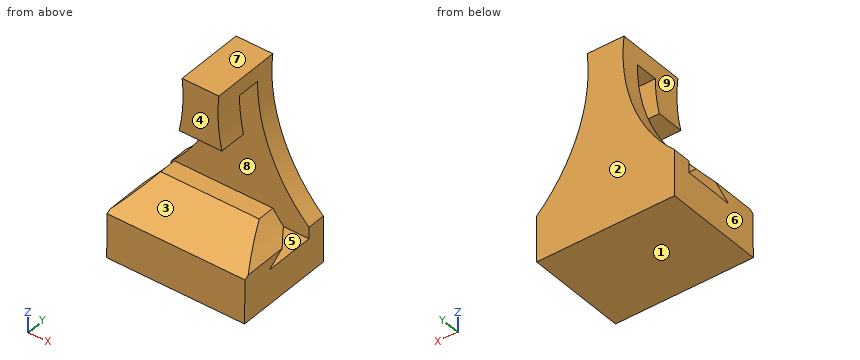
```python
from build123d import *

# Parameters (mm, degrees)
F1_DEPTH = 60
F3_DEPTH = 43.8751131995


# Not quite as in the source:
# - a pattern or mirror of a feature is missing from the dataset's text; its kind, count and spacing are read off the source's solid


with BuildPart() as f1:
    # F0 (on Right) → F1 (new body)
    with BuildSketch(Plane.YZ):
        Polygon((-43.8741131995, 0), (0, 0), (0, 80), (-30, 80), (-30, 56.7161887884), (-18, 56.7161887884), (-18, 72.701357305), (-8, 72.701357305), (-8, 15), (-30, 15), (-17.1229156852, 24.1054718941), (-17.1229156852, 29.8044607043), (-24.7526019812, 29.8044607043), (-43.619140311, 18.9982891026), align=None)
    extrude(amount=F1_DEPTH)

    # F2 (on face) → F3 (cut, through all)
    with BuildSketch(Plane(origin=(0, 0, 0), x_dir=(-1, 0, 0), z_dir=(0, 1, 0))):
        with BuildLine():
            Line((-60, 80), (-60, 20))
            ThreePointArc((-60, 20), (-42.0220624026, 47.4414228809), (-38, 80))
            Line((-38, 80), (-60, 80))
        make_face()
    f3 = extrude(amount=-F3_DEPTH, mode=Mode.SUBTRACT)

    # F3_copies: F3 across plane
    add(f3.mirror(Plane(origin=(30, 0, 0), x_dir=(0, 0, -1), z_dir=(-1, 0, 0))), mode=Mode.SUBTRACT)


solid = f1.part
```
Input: part model. Units: mm. Frame: model coordinates. Face numbers are marked on the shaded views. A direction names the side the tool comes from. Round coordinates to 2 decimals unless told otherwise and drop trailing zeros. Loops run counter-clockwise (first coordinate to the right, second up) from the corner with the lowest first, then second, coordinate; pieces in that order, holes last. Notation, with made-up numbers: (11, 8) - (16, 8) arc R34 cw to (16, 45) - close; hole circle Ø5 at (6.5, 65). An arc over 180 degrees is marked (long way). One line per item, written item: value. Start each with the question number.
(1) Draft query along Z for the marked faces 6, 7, 8 and 9. Return one class per face: +Z half, -Z half, draft (parallel to the pull), parting line (faces both ways), or undercut.
(2) Ray query, line 1 (Y direction, x = 34.5, z = 59.5); line 2 (Z direction, x = 19, y = -14); line 3 (Y direction, x = 40, z = 17). Return the intervals inside material, ascending. Write a range as [from, to].
(3) Section A-A, the plane y = -12. Return loops of the section in (x, z).
(4) Section D-D, the plane y = -37.5. Return loops of the section in (x, z).
(5) Section C-C, the plane y = -19. Return loops of the section in (x, z).
(6) Contact query for flat-ended pins moving along their axis: P1, Ø10, axis at y = -13.5, z = 28, coming from the -X side; P2, Ø15, axis at x = 31.5, z = 71.5, coming from the -Y side; P3, Ø4, axis at y = -22.5, z = 67.5, coming from the -X side; P4, Ø1, axis at y = -21, z = 20.5, coming from the +X side. Output: stop coordinate, or through.
(7) Access query for the marked faces 1, 2, 3, 4 and 5. Directions: +Z, -Z, +X, -X, +Y, -Y. A direction counts if a zero-diameter tool reaches every point of the face in a straight line with its end or side. Return the directions, or none.
(8) Section B-B, the plane x = 33. Return loops of the section in (y, z).
Results below:
1. face 6: draft
1. face 7: +Z half
1. face 8: undercut
1. face 9: undercut
2. line 1: [-30, -18], [-8, 0]
2. line 2: [0, 15]
2. line 3: [-43.65, -27.17], [-8, 0]
3. outline: (0, 0) - (60, 0) - (60, 15) - (0, 15) - close; (22, 80) arc R72.4 cw to (22.4, 72.7) - (37.6, 72.7) arc R72.4 cw to (38, 80) - close
4. outline: (0, 0) - (60, 0) - (60, 20) arc R72.4 cw to (57.5, 22.5) - (2.5, 22.5) arc R72.4 cw to (0, 20) - close
5. outline: (0, 0) - (60, 0) - (60, 15) - (0, 15) - close; (2.76, 22.78) - (57.24, 22.78) arc R72.4 cw to (51.43, 29.8) - (8.57, 29.8) arc R72.4 cw to start; (20.69, 56.72) - (39.31, 56.72) arc R72.4 cw to (38, 80) - (22, 80) arc R72.4 cw to start
6. P1: x = 4.37
6. P2: y = -30
6. P3: x = 22.08
6. P4: through
7. face 1: -Z, +X, -X, +Y, -Y
7. face 2: +Z, -Z, +X, -X, +Y
7. face 3: +X, -X, -Y
7. face 4: +Z, +X, -X, -Y
7. face 5: +X, -X
8. outline: (-43.87, 0) - (0, 0) - (0, 80) - (-30, 80) - (-30, 56.72) - (-18, 56.72) - (-18, 72.7) - (-8, 72.7) - (-8, 15) - (-30, 15) - (-17.12, 24.11) - (-17.12, 29.8) - (-24.75, 29.8) - (-43.62, 19) - close
